Model file for the job. Use its own axes, mm. Round coordinates to 2 decimals unless told otherwise and drop trailing zeros. Order: outer loops, then holes, each group sorted by start corner. A loop starts at its lowest first (then second) coordinate and runs counter-clockwise, first axis right, second up. Notation, with made-up numbers: (17.5, 8.25) - (65.5, 8.25) arc R12 ccw to (65.5, 25.25) - close; hole circle Ø11 at (-6.5, 79). An arc over 180 degrees is marked (long way). Put each result on its own line as item: value. Start each with the question number.
Item 1: Saw through at B-B on z = -9. List the corners of the cut face in (x, y).
Item 2: Pin check, flat tips, straight feed: pin 1 Ø12 at (x, z) = (-30, -5.5) entering from -Y; pin 2 Ø4 at (x, z) = (-19.5, -10) entering from -Y. Stop position of each tip, or through.
Item 3: Saw through at C-C on x = -21. List the corners of the cut face in (y, z).
Item 4: Saw through at D-D on x = -14.5. List the corners of the cut face in (y, z), plus the area to 3 significant figures.
Item 5: Probe probe 1 along Y at (x, z) = (-32, -11.5); probe 2 along Y at (x, z) = (-42, -15). List the from-to ranges inside material, lowest first.
Item 6: Saw through at A-A on y = 0.3. List the corners of the cut face in (x, z).
```python
from build123d import *

# Parameters (mm, degrees)
BOSS_EXTRU_1_DEPTH      = 20
BOSS_EXTRU_1_DEPTH_BACK = 20
ESQUISSE1_R             = 1
BOSS_EXTRU_2_DEPTH      = 40
ESQUISSE3_W             = 2.163419692
ESQUISSE3_H             = 2
BOSS_EXTRU_3_DEPTH      = 5
ESQUISSE4_W             = 2.163419692
ESQUISSE4_H             = 2
BOSS_EXTRU_4_DEPTH      = 5


with BuildPart() as part:
    # Esquisse1 → Boss.-Extru.1 (new, two sides: drawn at the far end of the back side and taken through both)
    with BuildSketch(Plane.XY.offset(-BOSS_EXTRU_1_DEPTH_BACK)):
        Circle(ESQUISSE1_R)
    extrude(amount=BOSS_EXTRU_1_DEPTH + BOSS_EXTRU_1_DEPTH_BACK)



with BuildPart() as body_2:
    # Esquisse2 → Boss.-Extru.2 (new body)
    with BuildSketch(Plane.XY.offset(20)):
        Polygon((-2.163419692, -1), (-62.163419692, 1), (-2.163419692, 1), align=None)
    extrude(amount=-BOSS_EXTRU_2_DEPTH)


with BuildPart() as part_1:
    add(part.part)

    add(body_2.part)  # Boss.-Extru.3 merges body 2
    # Esquisse3 → Boss.-Extru.3 (add)
    with BuildSketch(Plane.XY.offset(20)):
        with Locations((-1.081709846, 0)):
            Rectangle(ESQUISSE3_W, ESQUISSE3_H)
    extrude(amount=-BOSS_EXTRU_3_DEPTH)

    # Esquisse4 → Boss.-Extru.4 (add)
    with BuildSketch(Plane(origin=(0, 0, -20), x_dir=(-1, 0, 0), z_dir=(0, 0, -1))):
        with Locations((1.081709846, 0)):
            Rectangle(ESQUISSE4_W, ESQUISSE4_H)
    extrude(amount=-BOSS_EXTRU_4_DEPTH)


solid = part_1.part
```
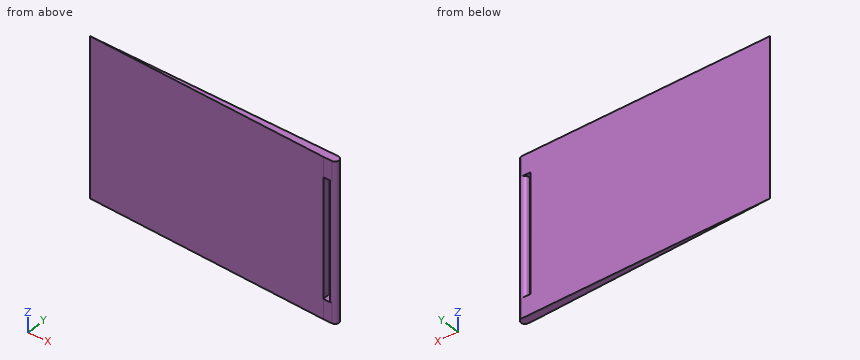
Results found:
1. outline: (-62.16, 1) - (-2.16, -1) - (-2.16, 1) - close; circle Ø2 at (0, 0)
2. pin 1: stops at y = -0.27
2. pin 2: stops at y = -0.49
3. outline: (-0.37, -20) - (1, -20) - (1, 20) - (-0.37, 20) - close
4. outline: (-0.59, -20) - (1, -20) - (1, 20) - (-0.59, 20) - close
4. area: 63.6 mm²
5. probe 1: y = -0.01 to 1
5. probe 2: y = 0.33 to 1
6. outline: (-41.16, -20) - (0.95, -20) - (0.95, 20) - (-41.16, 20) - close; hole (-2.16, -15) - (-0.95, -15) - (-0.95, 15) - (-2.16, 15) - close
